CAD build for the part. Positions are in the model's coordinates, mm. Coordinates: 2 decimals unless noted, no trailing zeros. Write each loop counter-clockwise with the first axis right and the second up, starting at its lowest first coordinate (ties: lowest second). Pieces come first, ordered by that corner, then holes.
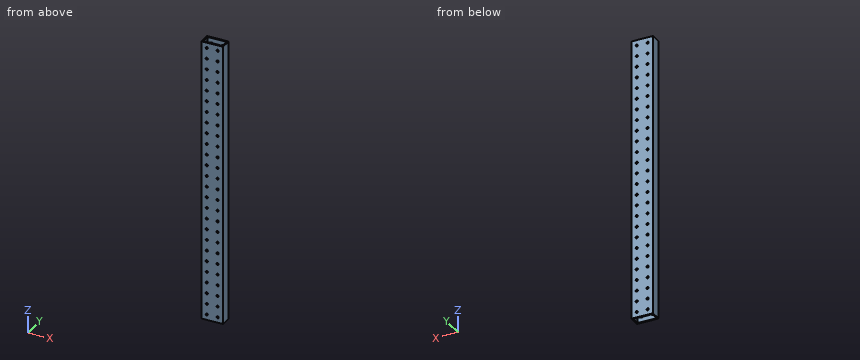
```python
from build123d import *

# Parameters (mm, degrees)
SKETCH1_W           = 50.8
SKETCH1_H           = 25.4
BOSS_EXTRUDE1_DEPTH = 660.4
SKETCH2_W           = 44.45
SKETCH2_H           = 19.05
CUT_EXTRUDE1_DEPTH  = 660.4
SKETCH3_R           = 2.54
CUT_EXTRUDE2_DEPTH  = 25.4


with BuildPart() as part:
    # Sketch1 → Boss-Extrude1 (new body)
    with BuildSketch(Plane.XY):
        with Locations((-12.7, -0.789265537)):
            Rectangle(SKETCH1_W, SKETCH1_H)
    extrude(amount=BOSS_EXTRUDE1_DEPTH)

    # Sketch2 → Cut-Extrude1 (cut)
    with BuildSketch(Plane.XY.offset(660.4)):
        with Locations((-12.7, -0.789265537)):
            Rectangle(SKETCH2_W, SKETCH2_H)
    extrude(amount=-CUT_EXTRUDE1_DEPTH, mode=Mode.SUBTRACT)

    # Sketch3 → Cut-Extrude2 (cut)
    with BuildSketch(Plane(origin=(0, 11.910734463, 0), x_dir=(1, 0, 0), z_dir=(0, 1, 0))):
        with Locations(Location((-25.4, -647.7, 0), (0, 0, 270))):
            Circle(SKETCH3_R)
        with Locations(Location((0, -647.7, 0), (0, 0, 270))):
            Circle(SKETCH3_R)
        with Locations(Location((0, -622.3, 0), (0, 0, 270))):
            Circle(SKETCH3_R)
        with Locations(Location((0, -596.9, 0), (0, 0, 270))):
            Circle(SKETCH3_R)
        with Locations(Location((0, -571.5, 0), (0, 0, 270))):
            Circle(SKETCH3_R)
        with Locations(Location((0, -546.1, 0), (0, 0, 270))):
            Circle(SKETCH3_R)
        with Locations(Location((0, -520.7, 0), (0, 0, 270))):
            Circle(SKETCH3_R)
        with Locations(Location((0, -495.3, 0), (0, 0, 270))):
            Circle(SKETCH3_R)
        with Locations(Location((0, -469.9, 0), (0, 0, 270))):
            Circle(SKETCH3_R)
        with Locations(Location((0, -444.5, 0), (0, 0, 270))):
            Circle(SKETCH3_R)
        with Locations(Location((0, -419.1, 0), (0, 0, 270))):
            Circle(SKETCH3_R)
        with Locations(Location((0, -393.7, 0), (0, 0, 270))):
            Circle(SKETCH3_R)
        with Locations(Location((0, -368.3, 0), (0, 0, 270))):
            Circle(SKETCH3_R)
        with Locations(Location((0, -342.9, 0), (0, 0, 270))):
            Circle(SKETCH3_R)
        with Locations(Location((0, -317.5, 0), (0, 0, 270))):
            Circle(SKETCH3_R)
        with Locations(Location((0, -292.1, 0), (0, 0, 270))):
            Circle(SKETCH3_R)
        with Locations(Location((0, -266.7, 0), (0, 0, 270))):
            Circle(SKETCH3_R)
        with Locations(Location((0, -241.3, 0), (0, 0, 270))):
            Circle(SKETCH3_R)
        with Locations(Location((0, -215.9, 0), (0, 0, 270))):
            Circle(SKETCH3_R)
        with Locations(Location((0, -190.5, 0), (0, 0, 270))):
            Circle(SKETCH3_R)
        with Locations(Location((0, -165.1, 0), (0, 0, 270))):
            Circle(SKETCH3_R)
        with Locations(Location((0, -139.7, 0), (0, 0, 270))):
            Circle(SKETCH3_R)
        with Locations(Location((0, -114.3, 0), (0, 0, 270))):
            Circle(SKETCH3_R)
        with Locations(Location((0, -88.9, 0), (0, 0, 270))):
            Circle(SKETCH3_R)
        with Locations(Location((0, -63.5, 0), (0, 0, 270))):
            Circle(SKETCH3_R)
        with Locations(Location((0, -38.1, 0), (0, 0, 270))):
            Circle(SKETCH3_R)
        with Locations(Location((0, -12.7, 0), (0, 0, 270))):
            Circle(SKETCH3_R)
        with Locations(Location((-25.4, -622.3, 0), (0, 0, 270))):
            Circle(SKETCH3_R)
        with Locations(Location((-25.4, -596.9, 0), (0, 0, 270))):
            Circle(SKETCH3_R)
        with Locations(Location((-25.4, -571.5, 0), (0, 0, 270))):
            Circle(SKETCH3_R)
        with Locations(Location((-25.4, -546.1, 0), (0, 0, 270))):
            Circle(SKETCH3_R)
        with Locations(Location((-25.4, -520.7, 0), (0, 0, 270))):
            Circle(SKETCH3_R)
        with Locations(Location((-25.4, -495.3, 0), (0, 0, 270))):
            Circle(SKETCH3_R)
        with Locations(Location((-25.4, -469.9, 0), (0, 0, 270))):
            Circle(SKETCH3_R)
        with Locations(Location((-25.4, -444.5, 0), (0, 0, 270))):
            Circle(SKETCH3_R)
        with Locations(Location((-25.4, -419.1, 0), (0, 0, 270))):
            Circle(SKETCH3_R)
        with Locations(Location((-25.4, -393.7, 0), (0, 0, 270))):
            Circle(SKETCH3_R)
        with Locations(Location((-25.4, -368.3, 0), (0, 0, 270))):
            Circle(SKETCH3_R)
        with Locations(Location((-25.4, -342.9, 0), (0, 0, 270))):
            Circle(SKETCH3_R)
        with Locations(Location((-25.4, -317.5, 0), (0, 0, 270))):
            Circle(SKETCH3_R)
        with Locations(Location((-25.4, -292.1, 0), (0, 0, 270))):
            Circle(SKETCH3_R)
        with Locations(Location((-25.4, -266.7, 0), (0, 0, 270))):
            Circle(SKETCH3_R)
        with Locations(Location((-25.4, -241.3, 0), (0, 0, 270))):
            Circle(SKETCH3_R)
        with Locations(Location((-25.4, -215.9, 0), (0, 0, 270))):
            Circle(SKETCH3_R)
        with Locations(Location((-25.4, -190.5, 0), (0, 0, 270))):
            Circle(SKETCH3_R)
        with Locations(Location((-25.4, -165.1, 0), (0, 0, 270))):
            Circle(SKETCH3_R)
        with Locations(Location((-25.4, -139.7, 0), (0, 0, 270))):
            Circle(SKETCH3_R)
        with Locations(Location((-25.4, -114.3, 0), (0, 0, 270))):
            Circle(SKETCH3_R)
        with Locations(Location((-25.4, -88.9, 0), (0, 0, 270))):
            Circle(SKETCH3_R)
        with Locations(Location((-25.4, -63.5, 0), (0, 0, 270))):
            Circle(SKETCH3_R)
        with Locations(Location((-25.4, -38.1, 0), (0, 0, 270))):
            Circle(SKETCH3_R)
        with Locations(Location((-25.4, -12.7, 0), (0, 0, 270))):
            Circle(SKETCH3_R)
    extrude(amount=-CUT_EXTRUDE2_DEPTH, mode=Mode.SUBTRACT)


solid = part.part
```
Item 1: Saw through at B-B, the plane y = -6.5. Write the cut outline in (x, z) (3 decimals), and give its area (3 significant figures).
Item 2: Wall check: line 1 along X through (y, z) = (9.6, 419.1); line 2 along Y through (x, z) = (-21, 79); line 3 along X through (y, z) = (0, 91.5) (3 decimals). Give the ranges that are in metal, low to high.
Item 3: Saw through at C-C, the plane z = 456.5. Write the cut outline in (x, y) (3 decimals).
Item 4: Saw through at A-A, the plane x = -11.5. Write the cut outline in (y, z), and give its area (3 significant figures).
Working result:
1. outline: (-38.1, 0) - (-34.925, 0) - (-34.925, 660.4) - (-38.1, 660.4) - close; (9.525, 0) - (12.7, 0) - (12.7, 660.4) - (9.525, 660.4) - close
1. area: 4,190 mm2
2. line 1: x = -38.1 to -27.94, -22.86 to -2.54, 2.54 to 12.7
2. line 2: y = -13.49 to -10.31, 8.74 to 11.91
2. line 3: x = -38.1 to -34.925, 9.525 to 12.7
3. outline: (-38.1, -13.489) - (12.7, -13.489) - (12.7, 11.911) - (-38.1, 11.911) - close; hole (-34.925, -10.314) - (9.525, -10.314) - (9.525, 8.736) - (-34.925, 8.736) - close
4. outline: (-13.49, 0) - (-10.31, 0) - (-10.31, 660.4) - (-13.49, 660.4) - close; (8.74, 0) - (11.91, 0) - (11.91, 660.4) - (8.74, 660.4) - close
4. area: 4,190 mm2
